Geometry: final body of the model. Coordinates: model frame, mm. A direction names the side the tool comes from. Give positions to 0.01 mm unless a question says otherwise; leave off trailing zeros. Write each loop counter-clockwise with the first axis right and the second up, starting at its lowest first coordinate (ties: lowest second). Pieces come first, ordered by that corner, then holes.
from build123d import *

# Parameters (mm, degrees)
SKETCH1_R           = 6
SKETCH1_R_2         = 1.7
BOSS_EXTRUDE1_DEPTH = 2
SKETCH2_W           = 2
SKETCH2_H           = 20.803847577
BOSS_EXTRUDE2_DEPTH = 2
SKETCH3_R           = 6
SKETCH3_R_2         = 1.7
BOSS_EXTRUDE3_DEPTH = 2
FILLET1_R           = 10


with BuildPart() as part:
    # Sketch1 → Boss-Extrude1 (new body)
    # profile 1 of 3: a face of its own
    with BuildSketch(Plane(origin=(0, 0, 0), x_dir=(1, 0, 0), z_dir=(0, 1, 0))):
        Circle(SKETCH1_R)
        with Locations(Location((0, 0, 0), (0, 0, 270))):
            Circle(SKETCH1_R_2, mode=Mode.SUBTRACT)
    # profile 2 of 3: a face of its own
    with BuildSketch(Plane(origin=(0, 0, 0), x_dir=(1, 0, 0), z_dir=(0, 1, 0))):
        with BuildLine():
            ThreePointArc((3, -5.196152423), (1.552914271, -5.795554958), (0, -6))
            Line((0, -6), (0, -26))
            Line((0, -26), (3, -26))
            Line((3, -26), (3, -5.196152423))
        make_face()
    # profile 3 of 3: a face of its own
    with BuildSketch(Plane(origin=(0, 0, 0), x_dir=(1, 0, 0), z_dir=(0, 1, 0))):
        with BuildLine():
            Line((0, -26), (0, -6))
            ThreePointArc((0, -6), (-1.552914271, -5.795554958), (-3, -5.196152423))
            Line((-3, -5.196152423), (-3, -26))
            Line((-3, -26), (0, -26))
        make_face()
    extrude(amount=BOSS_EXTRUDE1_DEPTH)

    # Sketch2 → Boss-Extrude2 (add)
    with BuildSketch(Plane(origin=(0, 2, 0), x_dir=(1, 0, 0), z_dir=(0, 1, 0))):
        with Locations((-2, -15.598076212)):
            Rectangle(SKETCH2_W, SKETCH2_H)
        with Locations((2, -15.598076212)):
            Rectangle(SKETCH2_W, SKETCH2_H)
    extrude(amount=BOSS_EXTRUDE2_DEPTH)

    # Sketch3 → Boss-Extrude3 (add)
    with BuildSketch(Plane(origin=(0, 2, 0), x_dir=(1, 0, 0), z_dir=(0, 1, 0))):
        Circle(SKETCH3_R)
        with Locations(Location((0, 0, 0), (0, 0, 270))):
            Circle(SKETCH3_R_2, mode=Mode.SUBTRACT)
    extrude(amount=BOSS_EXTRUDE3_DEPTH)

    # Fillet1
    fillet1_edges = [part.edges().sort_by_distance(p)[0] for p in [
        (-3, 2, 5.196152423),
        (3, 2, 5.196152423),
    ]]
    fillet(fillet1_edges, radius=FILLET1_R)


solid = part.part
Q1. Section C-C on x = 0. Output: boundary loops of the cut face in (y, z).
Filled sheet:
outline: (0, -6) - (4, -6) - (4, -1.7) - (0, -1.7) - close; (0, 1.7) - (4, 1.7) - (4, 6) - (2, 6) - (2, 26) - (0, 26) - close
Q2. Section B-B on y = 2.75. Output: boundary loops of the cut face in (x, z) (3 decimals), plus the area to 3 significant figures.
Filled sheet:
outline: (-4.875, 3.498) arc R6 ccw (long way) to (4.875, 3.498) arc R10 cw to (3, 9.327) - (3, 26) - (1, 26) - (1, 5.916) arc R6 ccw to (-1, 5.916) - (-1, 26) - (-3, 26) - (-3, 9.327) arc R10 cw to start; hole circle Ø3.4 at (0, 0)
area: 189 mm2
Q3. Section D-D on z = 10. Output: boundary loops of the cut face in (x, y).
Filled sheet:
outline: (-3, 0) - (3, 0) - (3, 4) - (1, 4) - (1, 2) - (-1, 2) - (-1, 4) - (-3, 4) - close
Q4. Access query for faces 4 (the flat face through (3, 2, 18)), 5 (the flat face through (-3, 2, 18)), 6 (the flat face through (-1, 3, 16)), 7 (the flat face through (1.2, 4, 9.8)). Directions: +Z, -Z, +X, -X, +Y, -Y. A direction counts if a zero-diameter tool reaches every point of the face in a straight line with its end or side. Return the directions, or none.
Filled sheet:
face 4: +Z, +X, +Y, -Y
face 5: +Z, -X, +Y, -Y
face 6: +Z, +Y
face 7: +Z, -Z, +X, -X, +Y
Q5. Section A-A on z = 0. Output: boundary loops of the cut face in (x, y), plus the area to 3 significant figures.
Filled sheet:
outline: (-6, 0) - (-1.7, 0) - (-1.7, 4) - (-6, 4) - close; (1.7, 0) - (6, 0) - (6, 4) - (1.7, 4) - close
area: 34.4 mm2
Q6. Pin query (flat end, axial travel): P1, Ø6, axis at x = 2, z = 15, coming from the -Y side; P2, Ø1, axis at y = 3, z = 13, coming from the +X side; P3, Ø2, axis at y = 1.5, z = 21.5, coming from the -X side; P4, Ø1.6, axis at x = 0, z = 21, coming from the +Y side. Return the tip coordinate at first contact, or that it passes through.
Filled sheet:
P1: stops at y = 0
P2: stops at x = 3
P3: stops at x = -3
P4: stops at y = 2
Q7. Pull-direction query (X, two-part tool) for faces 1 (the flat face through (0, 0, 10)), 2 (the cylindrical face through (0, 3, 6)), 3 (the cylindrical face through (-3.5, 2, 6.2)); classes: released by +X, released by -X, zero draft, split by the parting line, or undercut.
Filled sheet:
face 1: zero draft
face 2: undercut
face 3: released by -X
Q8. Ray query, line 1 along X through (y, z) = (2.2, 17); line 2 along X through (y, z) = (1.4, 0); line 3 along Z through (x, y) = (1, 0.75). Return the intervals inside material, ascending.
Filled sheet:
line 1: x = -3 to -1, 1 to 3
line 2: x = -6 to -1.7, 1.7 to 6
line 3: z = -5.92 to -1.37, 1.37 to 26
